Here's the drawing with two shaded views (mm, measured from the low corner). I have some questions. A direction names the side the tool comes from. Coordinates: 2 decimals unless noted, no trailing zeros. Write each loop counter-clockwise with the first axis right and the second up, starting at its lowest first coordinate (ties: lowest second). Pieces come first, ordered by that corner, then holes. Notation, with made-up numbers: (13.25, 0.25) -> (30.25, 0.25) arc R26 ccw to (30.25, 27.25) -> close; hole circle Ø4 at (81.25, -2). An arc over 180 degrees is marked (long way). Put each result on its own line as item: value.
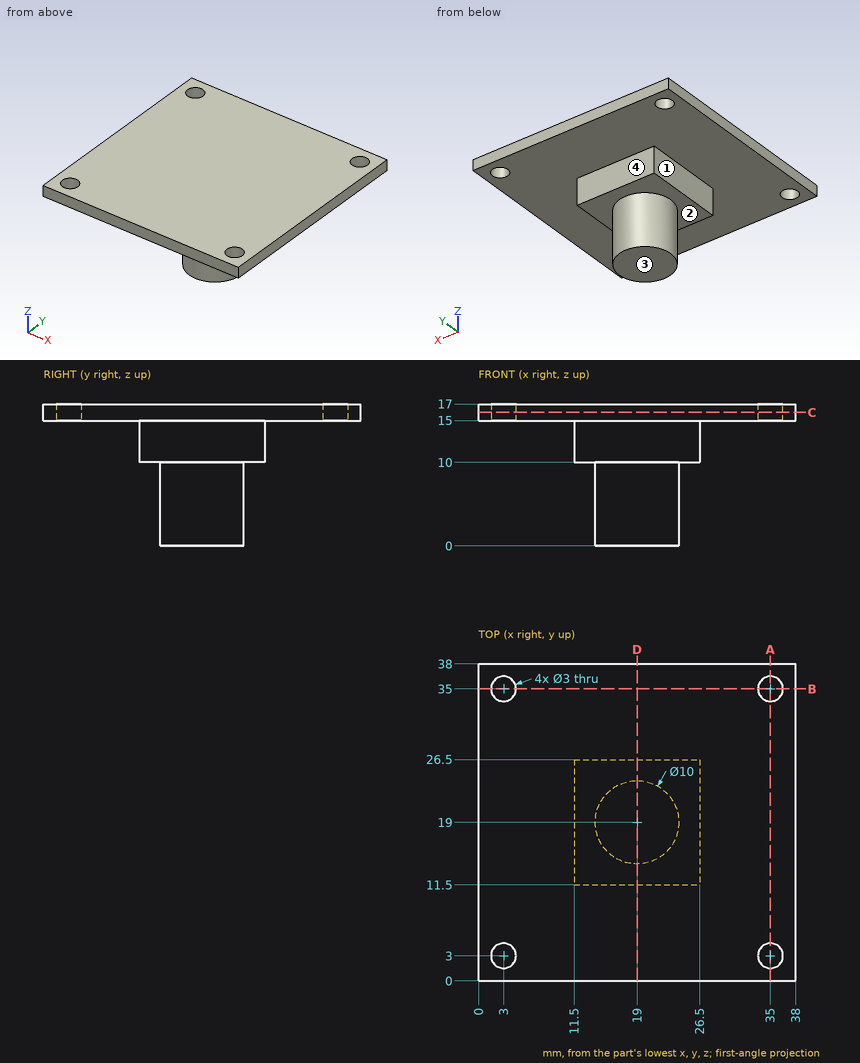
Item 1: Imagine slicing it at D-D on x = 19. Write out the boundary of the cut face in (y, z), then the cut area to 3 significant figures.
Output:
outline: (0, 15) -> (11.5, 15) -> (11.5, 10) -> (14, 10) -> (14, 0) -> (24, 0) -> (24, 10) -> (26.5, 10) -> (26.5, 15) -> (38, 15) -> (38, 17) -> (0, 17) -> close
area: 251 mm²
Item 2: Please list where these lines run through material, in increasing order: line 1 along Y through (x, z) = (3, 16.6); line 2 along Z through (x, y) = (5, 10.5); line 3 along Z through (x, y) = (14.5, 23). Write a range as from..to.
Output:
line 1: y = 0..1.5, 4.5..33.5, 36.5..38
line 2: z = 15..17
line 3: z = 10..17
Item 3: For P1, Ø4, axis at x = 31, y = 21, coming from the -Z side; P2, Ø1.5, axis at y = 22.5, z = 12, coming from the +X side; P3, Ø4.5, axis at x = 18, y = 20, coming from the -Z side; P4, Ø1.5, axis at x = 20.5, z = 13, coming from the -Y side, each with a flat end and sliding along its axis, tell me the tip position at first contact or that it passes through.
Output:
P1: stops at z = 15
P2: stops at x = 26.5
P3: stops at z = 0
P4: stops at y = 11.5
Item 4: Imagine slicing it at A-A on x = 35. Write out the boundary of the cut face in (y, z).
Output:
outline: (0, 15) -> (1.5, 15) -> (1.5, 17) -> (0, 17) -> close; (4.5, 15) -> (33.5, 15) -> (33.5, 17) -> (4.5, 17) -> close; (36.5, 15) -> (38, 15) -> (38, 17) -> (36.5, 17) -> close
Item 5: Which directions (+Z, -Z, +X, -X, +Y, -Y) give clear straight access to the entire face, cutting with the end or side of a thin tool? Please do the marked faces 1, 2, 3 and 4.
Output:
face 1: -Z, -X, +Y, -Y
face 2: -Z
face 3: -Z, +X, -X, +Y, -Y
face 4: -Z, +X, -X, +Y
Item 6: Imagine slicing it at C-C on z = 16. Write out the boundary of the cut face in (x, y).
Output:
outline: (0, 0) -> (38, 0) -> (38, 38) -> (0, 38) -> close; hole circle Ø3 at (3, 3); hole circle Ø3 at (3, 35); hole circle Ø3 at (35, 3); hole circle Ø3 at (35, 35)
